from build123d import *

# Parameters (mm, degrees)
CUT_EXTRUDE1_DEPTH = 1
CHAMFER1_SIZE      = 0.5
FILLET1_R          = 0.1
CHAMFER2_SIZE      = 0.2


with BuildPart() as part:
    # Sketch1 → Revolve1 (revolve)
    with BuildSketch(Plane(origin=(0, 0, 0), x_dir=(1, 0, 0), z_dir=(0, 1, 0))):
        Polygon((0, 3.604974233), (2.6, 3.604974233), (2.6, 3.104974233), (1.5, 2.004974233), (1.5, 0), (0, 0), align=None)
    revolve(axis=Axis((0, 0, 0), (0, 0, -1)))

    # Sketch2 → Cut-Extrude1 (cut)
    with BuildSketch(Plane(origin=(0, 0, -3.604974233), x_dir=(-1, 0, 0), z_dir=(0, 0, -1))):
        Polygon((1.5, 0), (0.75, 1.299038106), (-0.75, 1.299038106), (-1.5, 0), (-0.75, -1.299038106), (0.75, -1.299038106), align=None)
    extrude(amount=-CUT_EXTRUDE1_DEPTH, mode=Mode.SUBTRACT)

    # Chamfer1
    chamfer1_edges = [part.edges().sort_by_distance(p)[0] for p in [
        (-1.125, -0.649519053, -2.604974233),
        (0, -1.299038106, -2.604974233),
        (1.125, -0.649519053, -2.604974233),
        (1.125, 0.649519053, -2.604974233),
        (0, 1.299038106, -2.604974233),
        (-1.125, 0.649519053, -2.604974233),
    ]]
    chamfer(chamfer1_edges, length=CHAMFER1_SIZE)

    # Fillet1
    fillet1_edges = [part.edges().sort_by_distance(p)[0] for p in [
        (-1.5, 0, -2.004974233),
        (-2.6, 0, -3.104974233),
        (-2.6, 0, -3.604974233),
    ]]
    fillet(fillet1_edges, radius=FILLET1_R)

    # Chamfer2
    chamfer2_edges = [part.edges().sort_by_distance(p)[0] for p in [
        (-1.5, 0, 0),
    ]]
    chamfer(chamfer2_edges, length=CHAMFER2_SIZE)


solid = part.part
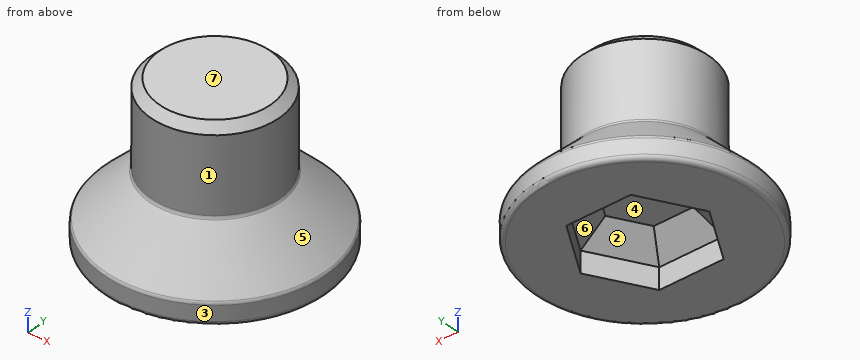
Here's how the part is built. I have some questions about the finished solid (model axes, mm). Face numbers are marked on the shaded views. A direction names the side the tool comes from. Give positions to 0.01 mm unless a question says otherwise; leave off trailing zeros. Order: outer loops, then holes, each group sorted by start corner. A loop starts at its lowest first (then second) coordinate and runs counter-clockwise, first axis right, second up. Notation, with made-up numbers: (62, 83.5) -> (98, 83.5) arc R18 ccw to (98, 118.5) -> close; hole circle Ø4 at (83.5, -11.5). An arc over 180 degrees is marked (long way). Use a Markdown table: item, result. Add a question column.
Item 1: Will these pins go through, and if not, where does the flat tip stop? pin 1 (1.5 mm diameter, centred on y = -2, z = -1, fed in from -X); pin 2 (1.8 mm diameter, centred on x = 0, y = 0, fed in from -Z); pin 3 (1.5 mm diameter, centred on y = -2, z = -2, fed in from -X).
Item 2: I need wall thicknesses on line 1 (Y direction, x = -0.05, z = -1.45); line 2 (Z direction, x = 0, y = -0.3); line 3 (X direction, y = 0.6, z = -2.85). Which ranges of each line are inside material? Lowest first, please.
Item 3: If we mould it in two halves opening along Y, with no side actions, what happens to the marked faces 4, 5, 6 and 7? For each: pulls with the +Y half, pulls with the -Y half, needs draft (parallel to the pull), parting line crosses it, or undercut.
Item 4: For the marked faces 1, 2 and 3, which set-ups out of +Z, -Z, +X, -X, +Y, -Y let a thin tool reach every point of the face, with its end or its side?
Item 5: Imagine slicing it at A-A on z = -0.4. Please give me the cut outline in (x, y), plus the area to 3 significant figures.
Data:
| question | item | result |
|---|---|---|
| 1 | pin 1 | stops at x = -0.83 |
| 1 | pin 2 | stops at z = -2.71 |
| 1 | pin 3 | stops at x = -1.41 |
| 2 | line 1 | y = -1.5 to 1.5 |
| 2 | line 2 | z = -2.6 to 0 |
| 2 | line 3 | x = -2.27 to -0.86, 0.86 to 2.27 |
| 3 | face 4 | undercut |
| 3 | face 5 | parting line crosses it |
| 3 | face 6 | undercut |
| 3 | face 7 | needs draft |
| 4 | face 1 | +Z |
| 4 | face 2 | -Z |
| 4 | face 3 | +Z, -Z |
| 5 | outline | circle Ø3 at (0, 0) |
| 5 | area | 7.07 mm² |
